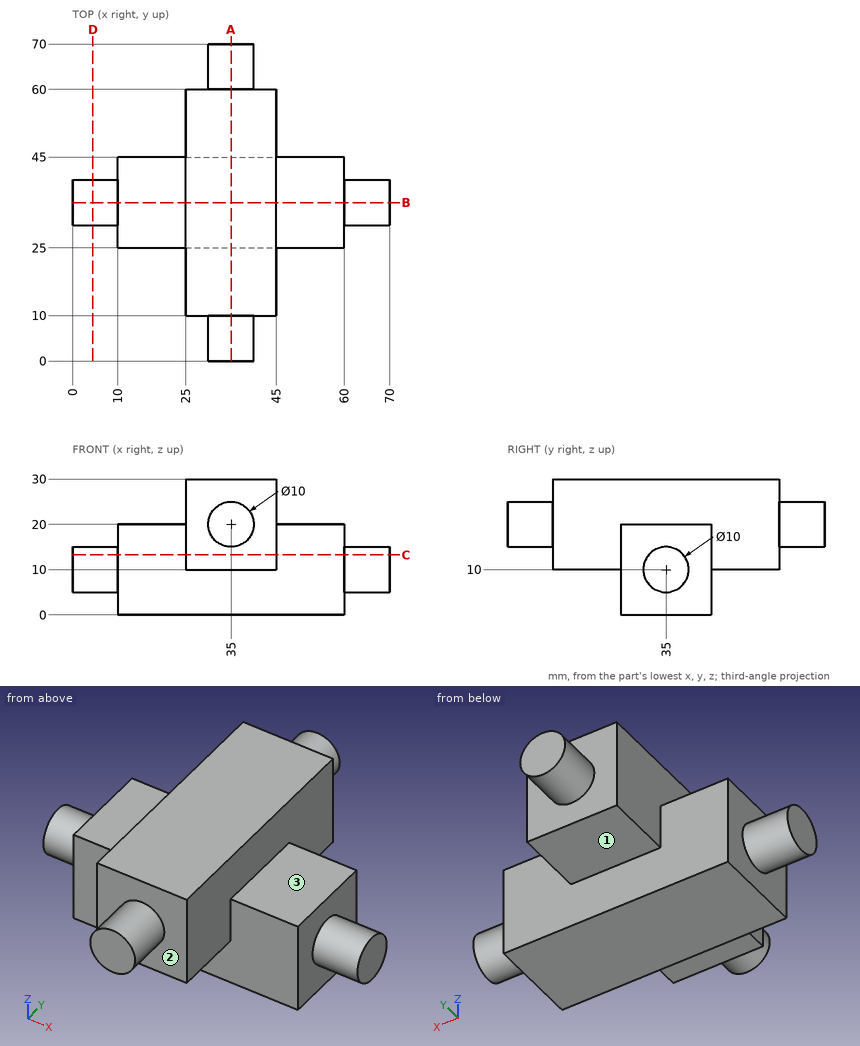
Study the drawing (mm; zero at the part's minimum x, y, z) and answer. A direction names the side the tool comes from. Coordinates: 2 decimals unless noted, no trailing zeros. Write each loop counter-clockwise with the first axis right and the second up, starting at its lowest first coordinate (ties: lowest second). Pieces come first, ordered by that corner, then holes. Notation, with made-up numbers: M 89,69.5 L 99,69.5 A24 cw 99,105.5 Z; hole C 15.25,-32.75 d6. An arc over 180 degrees is marked long. Use a Markdown table: item, result. Add a question column.
1. Straight lines are drawn through the part: line 1 along X through (y, z) = (40, 25.75); line 2 along Z through (x, y) = (16.5, 38). For each, find the intervals that lie inside material, in ascending order. Write a range as [from, to].
2. Section B-B (y = 35) is taken. Give the vertices of the cut face in (x, z), plus the area to 3 significant figures.
3. Section A-A (x = 35) is taken. Give the vertices of the cut face in (y, z).
4. Given P1, Ø4.5, axis at x = 54, y = 39.5, coming from the +Z side; P2, Ø1.5, axis at x = 60, z = 18.5, coming from the -Y side; P3, Ø12, axis at x = 34, y = 16.5, coming from the -Z side, each flat-ended and moving along its own axis, determine where each tip first touches the part or whether it passes through.
5. Section D-D (x = 4.5) is taken. Give the vertices of the cut face in (y, z), plus the area to 3 significant figures.
6. Section C-C (z = 13.25) is taken. Give the vertices of the cut face in (x, y), plus the area to 3 significant figures.
7. Which of the six approach directions +Z, -Z, +X, -X, +Y, -Y give full straight-line access (tool end or side, diameter ignored) to the marked faces 1, 2 and 3?
Data:
| question | item | result |
|---|---|---|
| 1 | line 1 | x = [25, 45] |
| 1 | line 2 | z = [0, 20] |
| 2 | outline | M 0,5 L 10,5 L 10,0 L 60,0 L 60,5 L 70,5 L 70,15 L 60,15 L 60,20 L 45,20 L 45,30 L 25,30 L 25,20 L 10,20 L 10,15 L 0,15 Z |
| 2 | area | 1,400 mm2 |
| 3 | outline | M 0,15 L 10,15 L 10,10 L 25,10 L 25,0 L 45,0 L 45,10 L 60,10 L 60,15 L 70,15 L 70,25 L 60,25 L 60,30 L 10,30 L 10,25 L 0,25 Z |
| 4 | P1 | stops at z = 20 |
| 4 | P2 | stops at y = 25 |
| 4 | P3 | stops at z = 10 |
| 5 | outline | C 35,10 d10 |
| 5 | area | 78.5 mm2 |
| 6 | outline | M 0,31.2 L 10,31.2 L 10,25 L 25,25 L 25,10 L 45,10 L 45,25 L 60,25 L 60,31.2 L 70,31.2 L 70,38.8 L 60,38.8 L 60,45 L 45,45 L 45,60 L 25,60 L 25,45 L 10,45 L 10,38.8 L 0,38.8 Z |
| 6 | area | 1,750 mm2 |
| 7 | face 1 | -Z, +X, -X, +Y |
| 7 | face 2 | -Y |
| 7 | face 3 | +Z, +X, +Y, -Y |
